Read the model definition and answer for the solid it produces. Units are mm, in the model's axes. Coordinates: 2 decimals unless noted, no trailing zeros. Order: outer loops, then holes, each group sorted by start corner. A loop starts at its lowest first (then second) coordinate and runs counter-clockwise, first axis right, second up. Notation, with made-up numbers: (18, 41.25) -> (76, 41.25) arc R22 cw to (76, 64.25) -> close; hole circle Ø10 at (24, 9.25). An arc over 180 degrees is marked (long way). Answer in a Markdown table with one row per item.
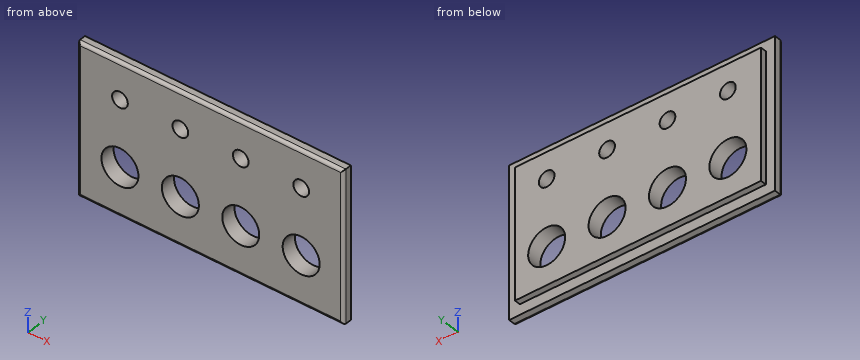
from build123d import *

# Parameters (mm, degrees)
SKETCH4_W               = 88
SKETCH4_H               = 50
BOSS_EXTRUDE2_DEPTH     = 3
SKETCH6_W               = 81.456613026
SKETCH6_H               = 43.073471677
BOSS_EXTRUDE3_DEPTH     = 2
CUT_EXTRUDE1_DEPTH      = 67.670833203
CUT_EXTRUDE1_DEPTH_BACK = 67.670833203
SKETCH5_R               = 6.125
SKETCH5_R_2             = 2.6
FILLET1_R               = 1


with BuildPart() as part:
    # Sketch4 → Boss-Extrude2 (new body)
    with BuildSketch(Plane(origin=(0, 0, 0), x_dir=(1, 0, 0), z_dir=(0, 1, 0))):
        with Locations((0, 25)):
            Rectangle(SKETCH4_W, SKETCH4_H)
    extrude(amount=BOSS_EXTRUDE2_DEPTH)

    # Sketch6 → Boss-Extrude3 (add)
    with BuildSketch(Plane(origin=(0, 3, 0), x_dir=(1, 0, 0), z_dir=(0, 1, 0))):
        with Locations((-0.228306513, 25.036735839)):
            Rectangle(SKETCH6_W, SKETCH6_H)
    extrude(amount=BOSS_EXTRUDE3_DEPTH)

    # Sketch5 → Cut-Extrude1 (cut, two sides: drawn at the far end of the back side and taken through both)
    with BuildSketch(Plane(origin=(0, 3, 0), x_dir=(-1, 0, 0), z_dir=(0, 1, 0)).offset(-CUT_EXTRUDE1_DEPTH_BACK)):
        with Locations(Location((-30, -34, 0), (0, 0, 90))):
            Circle(SKETCH5_R)
        with Locations(Location((-10, -34, 0), (0, 0, 90))):
            Circle(SKETCH5_R)
        with Locations(Location((10, -34, 0), (0, 0, 90))):
            Circle(SKETCH5_R)
        with Locations(Location((30, -34, 0), (0, 0, 90))):
            Circle(SKETCH5_R)
        with Locations(Location((-30, -12.206810763, 0), (0, 0, 90))):
            Circle(SKETCH5_R_2)
        with Locations(Location((-10, -12.206810763, 0), (0, 0, 90))):
            Circle(SKETCH5_R_2)
        with Locations(Location((10, -12.206810763, 0), (0, 0, 90))):
            Circle(SKETCH5_R_2)
        with Locations(Location((30, -12.206810763, 0), (0, 0, 90))):
            Circle(SKETCH5_R_2)
    extrude(amount=CUT_EXTRUDE1_DEPTH + CUT_EXTRUDE1_DEPTH_BACK, mode=Mode.SUBTRACT)

    # Fillet1
    fillet1_edges = [part.edges().sort_by_distance(p)[0] for p in [
        (0, 0, 0),
        (-44, 0, -25),
        (0, 0, -50),
        (44, 0, -25),
    ]]
    fillet(fillet1_edges, radius=FILLET1_R)


solid = part.part
Q1. Given pin 1 (1 mm diameter, centred on y = 4.5, z = -27, fed in from -X); pin 2 (16 mm diameter, centred on x = 10, z = -34, fed in from +Y); pin 3 (1 mm diameter, centred on x = -19, y = 4.5, fed in from +Z); pin 4 (1.6 mm diameter, centred on x = 16, y = 4, fed in from -Z), each flat-ended and moving along its own axis, determine where each tip first touches the part or whether it passes through.
Outcome:
| item | result |
|---|---|
| pin 1 | x = -40.96 |
| pin 2 | y = 5 |
| pin 3 | z = -3.5 |
| pin 4 | z = -46.57 |
Q2. The part is cut by section B-B (z = -5). Write down the section's boundary in (x, y).
Outcome:
| item | result |
|---|---|
| outline | (-44, 1) arc R1 ccw to (-43, 0) -> (43, 0) arc R1 ccw to (44, 1) -> (44, 3) -> (40.5, 3) -> (40.5, 5) -> (-40.96, 5) -> (-40.96, 3) -> (-44, 3) -> close |
Q3. Consider line 1 (X direction, y = 2, z = -34) (3 decimals); line 2 (Z direction, x = 30, y = 1.85) (3 decimals); line 3 (X direction, y = 2.7, z = -39). Determine where each line is inside the solid, lowest interval first.
Outcome:
| item | result |
|---|---|
| line 1 | -44 to -36.125, -23.875 to -16.125, -3.875 to 3.875, 16.125 to 23.875, 36.125 to 44 |
| line 2 | -50 to -40.125, -27.875 to -14.807, -9.607 to 0 |
| line 3 | -44 to -33.54, -26.46 to -13.54, -6.46 to 6.46, 13.54 to 26.46, 33.54 to 44 |
Q4. The part is cut by section D-D (z = -34). Write down the section's boundary in (x, y) (3 decimals).
Outcome:
| item | result |
|---|---|
| outline | (-44, 1) arc R1 ccw to (-43, 0) -> (-36.125, 0) -> (-36.125, 5) -> (-40.957, 5) -> (-40.957, 3) -> (-44, 3) -> close; (-23.875, 0) -> (-16.125, 0) -> (-16.125, 5) -> (-23.875, 5) -> close; (-3.875, 0) -> (3.875, 0) -> (3.875, 5) -> (-3.875, 5) -> close; (16.125, 0) -> (23.875, 0) -> (23.875, 5) -> (16.125, 5) -> close; (36.125, 0) -> (43, 0) arc R1 ccw to (44, 1) -> (44, 3) -> (40.5, 3) -> (40.5, 5) -> (36.125, 5) -> close |
Q5. The part is cut by section A-A (x = -30). Write down the section's boundary in (y, z) (3 decimals).
Outcome:
| item | result |
|---|---|
| outline | (0, -49) arc R1 ccw to (1, -50) -> (3, -50) -> (3, -46.573) -> (5, -46.573) -> (5, -40.125) -> (0, -40.125) -> close; (0, -27.875) -> (5, -27.875) -> (5, -14.807) -> (0, -14.807) -> close; (0, -9.607) -> (5, -9.607) -> (5, -3.5) -> (3, -3.5) -> (3, 0) -> (1, 0) arc R1 ccw to (0, -1) -> close |
Q6. The part is cut by section C-C (y = 2.15). Give the number of separate pieces and of enclosed holes in the cut face, then the cut area to 3 significant figures.
Outcome:
| item | result |
|---|---|
| separate pieces | 1 |
| enclosed holes | 8 |
| area | 3,840 mm² |
